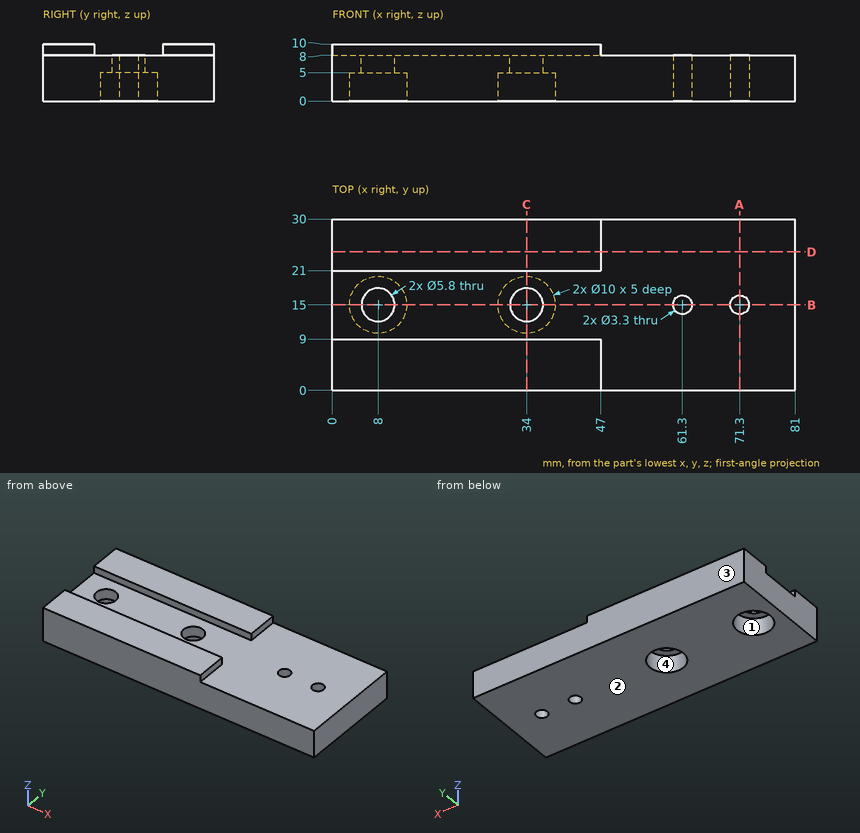
Answer from the drawing. Dimensions are ordinates in mm from the lowest x, y and z of the part. Give positions to 0.01 mm unless a question says otherwise; leave off trailing zeros. Order: outer loops, then holes, each group sorted by start corner. A loop starts at its lowest first (then second) coordinate and runs counter-clockwise, first axis right, second up. Notation, with made-up numbers: (80.5, 35) -> (118.5, 35) arc R8 ccw to (118.5, 41) -> close; hole circle Ø10 at (78.25, 26). An arc over 180 degrees is marked (long way). One line per item, written item: value.
Item 1: Find section B-B, the plane y = 15. Give the vertices of the cut face in (x, z).
Answer sheet:
outline: (0, 0) -> (3, 0) -> (3, 5) -> (5.1, 5) -> (5.1, 8) -> (0, 8) -> close; (10.9, 5) -> (13, 5) -> (13, 0) -> (29, 0) -> (29, 5) -> (31.1, 5) -> (31.1, 8) -> (10.9, 8) -> close; (36.9, 5) -> (39, 5) -> (39, 0) -> (59.65, 0) -> (59.65, 8) -> (36.9, 8) -> close; (62.95, 0) -> (69.65, 0) -> (69.65, 8) -> (62.95, 8) -> close; (72.95, 0) -> (81, 0) -> (81, 8) -> (72.95, 8) -> close
Item 2: Find section A-A, the plane x = 71.3. Give the vertices of the cut face in (y, z), plus the area to 3 significant figures.
Answer sheet:
outline: (0, 0) -> (13.35, 0) -> (13.35, 8) -> (0, 8) -> close; (16.65, 0) -> (30, 0) -> (30, 8) -> (16.65, 8) -> close
area: 214 mm²
Item 3: Find section C-C, the plane x = 34. Give the vertices of the cut face in (y, z), plus the area to 3 significant figures.
Answer sheet:
outline: (0, 0) -> (10, 0) -> (10, 5) -> (12.1, 5) -> (12.1, 8) -> (9, 8) -> (9, 10) -> (0, 10) -> close; (17.9, 5) -> (20, 5) -> (20, 0) -> (30, 0) -> (30, 10) -> (21, 10) -> (21, 8) -> (17.9, 8) -> close
area: 209 mm²
Item 4: Straight lines are drawn through the part: probe 1 along X at (y, z) = (14, 0.75); probe 2 along Y at (x, z) = (35, 9); probe 3 along Y at (x, z) = (34, 2.05). For each, find the intervals that lie inside material, in ascending order.
Answer sheet:
probe 1: 0 to 3.1, 12.9 to 29.1, 38.9 to 59.99, 62.61 to 69.99, 72.61 to 81
probe 2: 0 to 9, 21 to 30
probe 3: 0 to 10, 20 to 30
Item 5: Find section D-D, the plane y = 24.25. Give the vertices of the cut face in (x, z), plus the area to 3 significant figures.
Answer sheet:
outline: (0, 0) -> (81, 0) -> (81, 8) -> (47, 8) -> (47, 10) -> (0, 10) -> close
area: 742 mm²
Item 6: Flat-ended cylindrical pins translate along their axes: P1, Ø4.5, axis at x = 61.3, y = 15, coming from the +Z side; P2, Ø13, axis at x = 34, y = 15, coming from the -Z side; P3, Ø2, axis at y = 24, z = 9.5, coming from the +X side; P4, Ø2.5, axis at x = 71.3, y = 15, coming from the -Z side. Find the tip coordinate at first contact, or state that the pin passes through.
Answer sheet:
P1: z = 8
P2: z = 0
P3: x = 47
P4: through
Item 7: Determine the mould class of the marked faces 1, 2, 3 and 4 for opening direction Y: released by +Y, released by -Y, zero draft, split by the parting line, or undercut.
Answer sheet:
face 1: undercut
face 2: zero draft
face 3: released by +Y
face 4: undercut
